from build123d import *

# Parameters (mm, degrees)
BOSS_EXTRUDE1_DEPTH  = 3
SKETCH3_R            = 1.75
CUT_EXTRUDE2_DEPTH   = 4
LPATTERN1_COUNT      = 2
LPATTERN1_PITCH      = 70
LPATTERN1_COUNT_DIR2 = 2
LPATTERN1_PITCH_DIR2 = 90
SKETCH5_W            = 10
SKETCH5_H            = 10
CUT_EXTRUDE4_DEPTH   = 4


with BuildPart() as part:
    # Sketch1 → Boss-Extrude1 (new body)
    with BuildSketch(Plane(origin=(0, 0, 0), x_dir=(1, 0, 0), z_dir=(0, 1, 0))):
        with BuildLine():
            Line((-45, 40), (45, 40))
            ThreePointArc((45, 40), (48.535533906, 38.535533906), (50, 35))
            Line((50, 35), (50, -35))
            ThreePointArc((50, -35), (48.535533906, -38.535533906), (45, -40))
            Line((45, -40), (-45, -40))
            ThreePointArc((-45, -40), (-48.535533906, -38.535533906), (-50, -35))
            Line((-50, -35), (-50, 35))
            ThreePointArc((-50, 35), (-48.535533906, 38.535533906), (-45, 40))
        make_face()
    extrude(amount=BOSS_EXTRUDE1_DEPTH)

    # Sketch3 → Cut-Extrude2 (cut, through all)
    with BuildSketch(Plane(origin=(0, 3, 0), x_dir=(1, 0, 0), z_dir=(0, 1, 0))):
        with Locations((-45, -35)):
            Circle(SKETCH3_R)
    cut_extrude2 = extrude(amount=-CUT_EXTRUDE2_DEPTH, mode=Mode.SUBTRACT)

    # LPattern1: Cut-Extrude2 2 × 2
    with Locations(*[(j * LPATTERN1_PITCH_DIR2, 0, -i * LPATTERN1_PITCH) for i in range(LPATTERN1_COUNT) for j in range(LPATTERN1_COUNT_DIR2) if (i, j) != (0, 0)]):
        add(cut_extrude2, mode=Mode.SUBTRACT)

    # Sketch5 → Cut-Extrude4 (cut, through all)
    with BuildSketch(Plane(origin=(0, 3, 0), x_dir=(1, 0, 0), z_dir=(0, 1, 0))):
        with Locations((-35, -35)):
            Rectangle(SKETCH5_W, SKETCH5_H)
        with Locations((35, 35)):
            Rectangle(SKETCH5_W, SKETCH5_H)
    extrude(amount=-CUT_EXTRUDE4_DEPTH, mode=Mode.SUBTRACT)


solid = part.part
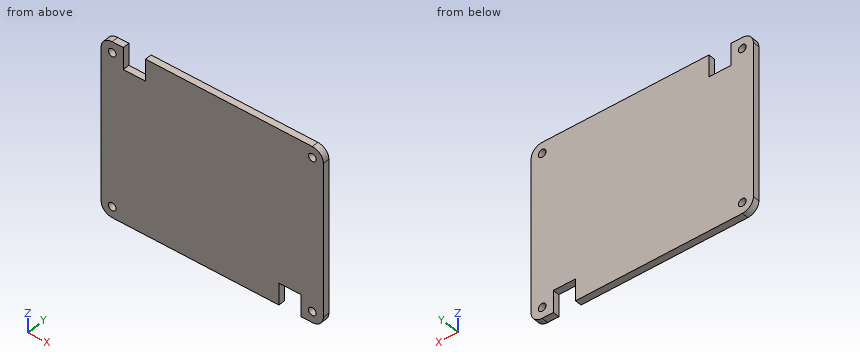
Work out the finished part from the listing and answer in its coordinate system (mm). Round coordinates to 2 decimals unless told otherwise and drop trailing zeros. Write each loop counter-clockwise with the first axis right and the second up, starting at its lowest first coordinate (ties: lowest second). Pieces come first, ordered by that corner, then holes. Notation, with made-up numbers: (40.25, -34.75) -> (48.25, -34.75) arc R30 ccw to (48.25, 2.25) -> close; hole circle Ø11 at (-16, 81). An arc over 180 degrees is marked (long way). Answer as CSV lines item,"result". Start each with the question number.
(1) The part is cut by section B-B, the plane y = 1.6. Give the vertices of the cut face in (x, z), then the cut area to 3 significant figures.
(2) The part is cut by section A-A, the plane z = 32. Give the vertices of the cut face in (x, y).
(3) The part is cut by section C-C, the plane x = 35.5. Give the vertices of the cut face in (y, z).
(4) Each of these flat-tipped pins is pushed along its axis until it touches: pin 1 (2 mm diameter, centred on x = -45, z = -35, fed in from +Y); pin 2 (1 mm diameter, centred on x = -37, y = 0.5, fed in from +Z). Where does it stop, or does it pass through?
(5) Find the intervals of material crossed by probe 1 along Z at (x, y) = (-45, 1.85); probe 2 along X at (y, z) = (1.05, -35); probe 3 along X at (y, z) = (1.65, 35), in increasing order.
Output values:
1,outline,"(-50, -35) arc R5 ccw to (-45, -40) -> (30, -40) -> (30, -30) -> (40, -30) -> (40, -40) -> (45, -40) arc R5 ccw to (50, -35) -> (50, 35) arc R5 ccw to (45, 40) -> (-30, 40) -> (-30, 30) -> (-40, 30) -> (-40, 40) -> (-45, 40) arc R5 ccw to (-50, 35) -> close; hole circle Ø3.5 at (-45, -35); hole circle Ø3.5 at (-45, 35); hole circle Ø3.5 at (45, -35); hole circle Ø3.5 at (45, 35)"
1,area,"7,740 mm²"
2,outline,"(-50, 0) -> (-40, 0) -> (-40, 3) -> (-50, 3) -> close; (-30, 0) -> (50, 0) -> (50, 3) -> (-30, 3) -> close"
3,outline,"(0, -30) -> (3, -30) -> (3, 40) -> (0, 40) -> close"
4,pin 1,"passes through"
4,pin 2,"stops at z = 30"
5,probe 1,"z = -40 to -36.75, -33.25 to 33.25, 36.75 to 40"
5,probe 2,"x = -50 to -46.75, -43.25 to 30, 40 to 43.25, 46.75 to 50"
5,probe 3,"x = -50 to -46.75, -43.25 to -40, -30 to 43.25, 46.75 to 50"
